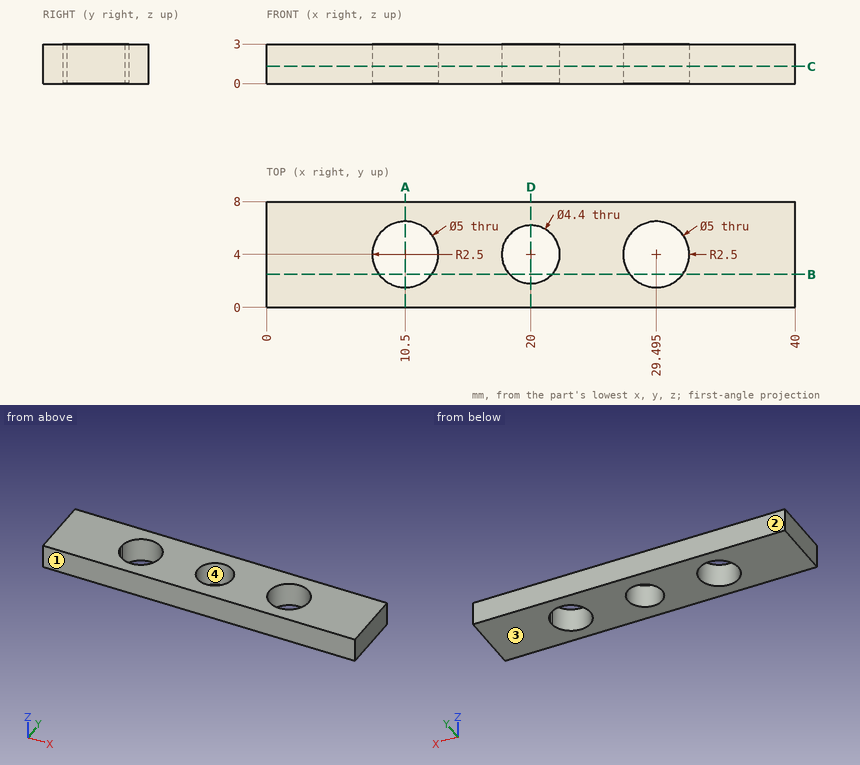
Design review of the part shown in the three views and the two pictorial views. Dimensions are in mm from the part's minimum x, y and z. Coordinates: 2 decimals unless noted, no trailing zeros. Loops run counter-clockwise (first coordinate to the right, second up) from the corner with the lowest first, then second, coordinate; pieces in that order, holes last. Notation, with made-up numbers: (46.25, 27.5) -> (50.25, 27.5) arc R25 ccw to (50.25, 61.5) -> close; hole circle Ø7 at (67, 13.25). An arc over 180 degrees is marked (long way). Answer as CSV lines item,"result".
Item 1: Draft analysis for pull direction Y (two halves, no side actions). For the marked faces 1, 2, 3 and 4, state which applies: +Y half, -Y half, draft (parallel to the pull), parting line (faces both ways), or undercut.
Results below:
face 1,"-Y half"
face 2,"+Y half"
face 3,"draft"
face 4,"undercut"
Item 2: For L1, parallel to Y at x = 10.5, z = 1.35; L2, parallel to Y at x = 20, z = 0.1; L3, parallel to X at y = 3.25, z = 0.9 (1 decimal), list the stretches that pass through material, from the lowest coordinate up.
Results below:
L1,"y = 0 to 1.5, 6.5 to 8"
L2,"y = 0 to 1.8, 6.2 to 8"
L3,"x = 0 to 8.1, 12.9 to 17.9, 22.1 to 27.1, 31.9 to 40"
Item 3: Take a section at B-B, the plane y = 2.5. State the section outline as (x, z) points (1 decimal).
Results below:
outline,"(0, 0) -> (8.5, 0) -> (8.5, 3) -> (0, 3) -> close; (12.5, 0) -> (18.4, 0) -> (18.4, 3) -> (12.5, 3) -> close; (21.6, 0) -> (27.5, 0) -> (27.5, 3) -> (21.6, 3) -> close; (31.5, 0) -> (40, 0) -> (40, 3) -> (31.5, 3) -> close"
Item 4: Take a section at D-D, the plane x = 20. State the section outline as (y, z) points.
Results below:
outline,"(0, 0) -> (1.8, 0) -> (1.8, 3) -> (0, 3) -> close; (6.2, 0) -> (8, 0) -> (8, 3) -> (6.2, 3) -> close"
Item 5: Insertion check: pin 1 (1 mm diameter, centred on y = 2, z = 2, fed in from -X). The pin has a flat end and moves straight along its axis. Give the tip position at first contact, or say it passes through.
Results below:
pin 1,"stops at x = 0"
Item 6: Take a section at A-A, the plane x = 10.5. State the section outline as (y, z) points.
Results below:
outline,"(0, 0) -> (1.5, 0) -> (1.5, 3) -> (0, 3) -> close; (6.5, 0) -> (8, 0) -> (8, 3) -> (6.5, 3) -> close"
Item 7: Take a section at C-C, the plane z = 1.3. Count the separate pieces of the cut face and the enclosed holes in it.
Results below:
separate pieces,"1"
enclosed holes,"3"
